Geometry: final body of the model. Coordinates: model frame, mm. A direction names the side the tool comes from. Give positions to 0.01 mm unless a question says otherwise; leave off trailing zeros. Loops run counter-clockwise (first coordinate to the right, second up) from the corner with the lowest first, then second, coordinate; pieces in that order, holes last. Notation, with made-up numbers: (-25.5, 82) -> (31.5, 82) arc R16 ccw to (31.5, 91) -> close; hole circle Ø10 at (68, 0.25). An arc over 180 degrees is marked (long way). One line per item, written item: value. Start each with the question number.
from build123d import *

# Parameters (mm, degrees)
EXTRUDE_1_DEPTH     = 40
SKETCH_1_3_W        = 33.7
SKETCH_1_3_H        = 20
EXTRUDE_2_DEPTH     = 4
SKETCH_2_W          = 51.7
SKETCH_2_H          = 49
EXTRUDE_3_DEPTH     = 4
SKETCH_3_R          = 4
CUT_EXTRUDE_1_DEPTH = 8


with BuildPart() as part:
    # Sketch 1 → Extrude 1 (new body)
    with BuildSketch(Plane.XY):
        Polygon((16.85, -13), (20.85, -13), (20.85, 13), (-20.85, 13), (-20.85, -13), (-16.85, -13), (-16.85, 7), (16.85, 7), align=None)
    extrude(amount=EXTRUDE_1_DEPTH)

    # Sketch 1_3 → Extrude 2 (add)
    with BuildSketch(Plane.XY):
        with Locations((0, -3)):
            Rectangle(SKETCH_1_3_W, SKETCH_1_3_H)
        Polygon((16.85, -13), (20.85, -13), (20.85, 13), (-20.85, 13), (-20.85, -13), (-16.85, -13), (-16.85, 7), (16.85, 7), align=None)
    extrude(amount=-EXTRUDE_2_DEPTH)

    # Sketch 2 → Extrude 3 (add)
    with BuildSketch(Plane(origin=(0, 13, 0), x_dir=(1, 0, 0), z_dir=(0, 1, 0))):
        with Locations((0, -15.5)):
            Rectangle(SKETCH_2_W, SKETCH_2_H)
    extrude(amount=-EXTRUDE_3_DEPTH)

    # Sketch 3 → Cut-Extrude 1 (cut)
    with BuildSketch(Plane.XZ.offset(-7)):
        with Locations(Location((0, 13.75, 0), (0, 0, 270))):
            Circle(SKETCH_3_R)
    extrude(amount=-CUT_EXTRUDE_1_DEPTH, mode=Mode.SUBTRACT)


solid = part.part
Item 1: Mould query, pull axis X, two halves, no side actions, for faces 6 (the face through (-16.85, -3, 20)), 7 (the face through (-2, 9, -5)), 8 (the face through (-25.85, 11, 16)). Classes: pulls with the +X half, pulls with the -X half, needs draft (parallel to the pull), parting line crosses it, or undercut.
Item 2: Section D-D, the plane y = -5. Output: boundary loops of the cut face in (x, z), then the cut area to 3 significant figures.
Item 3: Access query for faces 1 (the face through (16.85, -3, 20)), 2 (the face through (20.85, -2, 18)), 3 (the face through (0, 9, 40)), 4 (the face through (-20.85, -2, 18)), 5 (the face through (0, -2, -4)). Directions: +Z, -Z, +X, -X, +Y, -Y. A direction counts if a zero-diameter tool reaches every point of the face in a straight line with its end or side. Return the directions, or none.
Item 4: Pin query (flat end, axial travel): pin 1 (4 mm diameter, centred on x = -0.5, y = -10, fed in from +Z); pin 2 (10 mm diameter, centred on y = -0.5, z = 7.5, fed in from -X); pin 3 (5 mm diameter, centred on y = -4.5, z = 18, fed in from +X). Return the tip coordinate at first contact, or that it passes through.
Item 5: Section B-B, the plane x = 0. Output: boundary loops of the cut face in (y, z), then the cut area to 3 significant figures.
Item 6: Section C-C, the plane z = 22. Output: boundary loops of the cut face in (x, y), then the cut area to 3 significant figures.
Item 7: Ray query, line 1 along X through (y, z) = (10.9, 13.75); line 2 along X through (y, z) = (-3, 12.5); line 3 along Z through (x, y) = (20.5, -8.25). Return the intervals inside material, ascending. Write a range as [from, to].
Item 8: Section A-A, the plane z = 13.75. Output: boundary loops of the cut face in (x, y), then the cut area to 3 significant figures.
Geometry check:
1. face 6: undercut
1. face 7: needs draft
1. face 8: pulls with the -X half
2. outline: (-20.85, -4) -> (20.85, -4) -> (20.85, 40) -> (16.85, 40) -> (16.85, 0) -> (-16.85, 0) -> (-16.85, 40) -> (-20.85, 40) -> close
2. area: 487 mm2
3. face 1: +Z, -Y
3. face 2: +Z, -Z, +X, -Y
3. face 3: +Z, +X, -X, +Y, -Y
3. face 4: +Z, -Z, -X, -Y
3. face 5: -Z, +X, -X, -Y
4. pin 1: stops at z = 0
4. pin 2: stops at x = -20.85
4. pin 3: stops at x = 20.85
5. outline: (-13, -4) -> (9, -4) -> (9, -9) -> (13, -9) -> (13, 9.75) -> (7, 9.75) -> (7, 0) -> (-13, 0) -> close; (7, 17.75) -> (13, 17.75) -> (13, 40) -> (7, 40) -> close
5. area: 316 mm2
6. outline: (-25.85, 9) -> (-20.85, 9) -> (-20.85, -13) -> (-16.85, -13) -> (-16.85, 7) -> (16.85, 7) -> (16.85, -13) -> (20.85, -13) -> (20.85, 9) -> (25.85, 9) -> (25.85, 13) -> (-25.85, 13) -> close
6. area: 450 mm2
7. line 1: x = [-25.85, -4], [4, 25.85]
7. line 2: x = [-20.85, -16.85], [16.85, 20.85]
7. line 3: z = [-4, 40]
8. outline: (-25.85, 9) -> (-20.85, 9) -> (-20.85, -13) -> (-16.85, -13) -> (-16.85, 7) -> (-4, 7) -> (-4, 13) -> (-25.85, 13) -> close; (4, 7) -> (16.85, 7) -> (16.85, -13) -> (20.85, -13) -> (20.85, 9) -> (25.85, 9) -> (25.85, 13) -> (4, 13) -> close
8. area: 402 mm2
